from build123d import *

# Parameters (mm, degrees)
EXTRUDE_1_DEPTH     = 48
SKETCH_3_W          = 2
SKETCH_3_H          = 3.503465233
EXTRUDE_2_DEPTH     = 0.5
SKETCH_4_W          = 2
SKETCH_4_H          = 3.503465233
EXTRUDE_3_DEPTH     = 0.5
SKETCH_7_W          = 0.5
SKETCH_7_H          = 3.503465233
CUT_EXTRUDE_2_DEPTH = 66.5
SKETCH_10_W         = 2
SKETCH_10_H         = 0.5
CUT_EXTRUDE_3_DEPTH = 66.5
SKETCH_13_W         = 0.5
SKETCH_13_H         = 2
SKETCH_16_W         = 0.5
SKETCH_16_H         = 2


with BuildPart() as part:
    # Эскиз1 → Бобышка-Вытянуть1 (new body)
    with BuildSketch(Plane.XY):
        with BuildLine():
            Line((0.5, 0), (0.5, 25.5))
            ThreePointArc((0.5, 25.5), (0.646446609, 25.853553391), (1, 26))
            Line((1, 26), (18.5, 26))
            ThreePointArc((18.5, 26), (18.853553391, 25.853553391), (19, 25.5))
            Line((19, 25.5), (19, 0))
            Line((19, 0), (19.5, 0))
            Line((19.5, 0), (19.5, 25.5))
            ThreePointArc((19.5, 25.5), (19.207106781, 26.207106781), (18.5, 26.5))
            Line((18.5, 26.5), (1, 26.5))
            ThreePointArc((1, 26.5), (0.292893219, 26.207106781), (0, 25.5))
            Line((0, 25.5), (0, 0))
            Line((0, 0), (0.5, 0))
        make_face()
    extrude(amount=EXTRUDE_1_DEPTH)

    # Эскиз3 → Бобышка-Вытянуть2 (add)
    with BuildSketch(Plane.ZY):
        with Locations((45, -1.751732617)):
            Rectangle(SKETCH_3_W, SKETCH_3_H)
        with Locations((3, -1.751732617)):
            Rectangle(SKETCH_3_W, SKETCH_3_H)
    extrude(amount=-EXTRUDE_2_DEPTH)

    # Эскиз4 → Бобышка-Вытянуть3 (add)
    with BuildSketch(Plane(origin=(19.5, 0, 0), x_dir=(0, 0, -1), z_dir=(1, 0, 0))):
        with Locations((-45, -1.751732617)):
            Rectangle(SKETCH_4_W, SKETCH_4_H)
        with Locations((-3, -1.751732617)):
            Rectangle(SKETCH_4_W, SKETCH_4_H)
    extrude(amount=-EXTRUDE_3_DEPTH)

    # Эскиз7 → Вырез-Вытянуть2 (cut)
    with BuildSketch(Plane.ZY):
        with Locations((45.75, -1.751732617)):
            Rectangle(SKETCH_7_W, SKETCH_7_H)
        with Locations((3.75, -1.751732617)):
            Rectangle(SKETCH_7_W, SKETCH_7_H)
        with Locations((44.25, -1.751732617)):
            Rectangle(SKETCH_7_W, SKETCH_7_H)
        with Locations((2.25, -1.751732617)):
            Rectangle(SKETCH_7_W, SKETCH_7_H)
    extrude(amount=-CUT_EXTRUDE_2_DEPTH, mode=Mode.SUBTRACT)

    # По траектории2: sweep along a path in Эскиз9
    with BuildLine(Plane.ZY) as sweep_2_path:
        Line((48, 24.75), (48.353553391, 25.103553391))
        ThreePointArc((48.353553391, 25.103553391), (48.461939766, 25.265765065), (48.5, 25.457106781))
        Line((48.5, 25.457106781), (48.5, 25.75))
        ThreePointArc((48.5, 25.75), (48.353553391, 26.103553391), (48, 26.25))
        Line((48, 26.25), (0, 26.25))
        ThreePointArc((0, 26.25), (-0.353553391, 26.103553391), (-0.5, 25.75))
        Line((-0.5, 25.75), (-0.5, 25.457106781))
        ThreePointArc((-0.5, 25.457106781), (-0.461939766, 25.265765065), (-0.353553391, 25.103553391))
        Line((-0.353553391, 25.103553391), (0, 24.75))
    # Эскиз10 → По траектории2 (sweep)
    with BuildSketch(Plane(origin=(0, 24.75, 48), x_dir=(1, 0, 0), z_dir=(0, 0.7071067811865477, 0.7071067811865475))):
        with Locations((9.75, 0)):
            Rectangle(SKETCH_10_W, SKETCH_10_H)
    sweep(path=sweep_2_path.line)

    # Эскиз14 → Вырез-Вытянуть3 (cut)
    with BuildSketch(Plane.ZY):
        Polygon((2.5, 0), (3.5, 0), (3.5, 3), (44.5, 3), (44.5, 0), (45.5, 0), (45.5, 3), (48, 3), (48, 0), (46.949999013, 0), (46.949999013, -4.072410454), (1.67699977, -4.072410454), (1.67699977, 0), (0, 0), (0, 3), (2.5, 3), align=None)
    extrude(amount=-CUT_EXTRUDE_3_DEPTH, mode=Mode.SUBTRACT)

    # По траектории3: sweep along a path in Эскиз11
    with BuildLine(Plane(origin=(0, 26.5, 0), x_dir=(1, 0, 0), z_dir=(0, 1, 0))) as sweep_3_path:
        Line((17.75, 0), (18.103553391, 0.353553391))
        ThreePointArc((18.103553391, 0.353553391), (18.265765065, 0.461939766), (18.457106781, 0.5))
        Line((18.457106781, 0.5), (18.75, 0.5))
        ThreePointArc((18.75, 0.5), (19.103553391, 0.353553391), (19.25, 0))
        Line((19.25, 0), (19.25, -48))
        ThreePointArc((19.25, -48), (19.103553391, -48.353553391), (18.75, -48.5))
        Line((18.75, -48.5), (18.457106781, -48.5))
        ThreePointArc((18.457106781, -48.5), (18.265765065, -48.461939766), (18.103553391, -48.353553391))
        Line((18.103553391, -48.353553391), (17.75, -48))
    # Эскиз13 → По траектории3 (sweep)
    with BuildSketch(Plane(origin=(17.75, 26.5, 0), x_dir=(0.7071067811865498, 0, 0.7071067811865454), z_dir=(-0.7071067811865454, 0, 0.7071067811865498))):
        with Locations((0, -13.25)):
            Rectangle(SKETCH_13_W, SKETCH_13_H)
    sweep(path=sweep_3_path.line)

    # По траектории4: sweep along a path in Эскиз15
    with BuildLine(Plane(origin=(0, 26.5, 0), x_dir=(1, 0, 0), z_dir=(0, 1, 0))) as sweep_4_path:
        Line((1.75, 0), (1.396446609, 0.353553391))
        ThreePointArc((1.396446609, 0.353553391), (1.234234935, 0.461939766), (1.042893219, 0.5))
        Line((1.042893219, 0.5), (0.75, 0.5))
        ThreePointArc((0.75, 0.5), (0.396446609, 0.353553391), (0.25, 0))
        Line((0.25, 0), (0.25, -48))
        ThreePointArc((0.25, -48), (0.396446609, -48.353553391), (0.75, -48.5))
        Line((0.75, -48.5), (1.042893219, -48.5))
        ThreePointArc((1.042893219, -48.5), (1.234234935, -48.461939766), (1.396446609, -48.353553391))
        Line((1.396446609, -48.353553391), (1.75, -48))
    # Эскиз16 → По траектории4 (sweep)
    with BuildSketch(Plane(origin=(1.75, 26.5, 48), x_dir=(-0.7071067811865488, 0, -0.7071067811865464), z_dir=(0.7071067811865464, 0, -0.7071067811865488))):
        with Locations((0, -13.25)):
            Rectangle(SKETCH_16_W, SKETCH_16_H)
    sweep(path=sweep_4_path.line)


solid = part.part
Can you work these out from the model? Positions are in its coordinate system, mm. A direction names the side the tool comes from. Round coordinates to 2 decimals unless told otherwise and drop trailing zeros. Write each loop counter-clockwise with the first axis right and the second up, starting at its lowest first coordinate (ties: lowest second). Pieces come first, ordered by that corner, then holes. Notation, with made-up numbers: M 6,-7 L 17,-7 A21 cw 17,15 Z; hole C 77.5,17 d4. An arc over 180 degrees is marked long. Use a Markdown table: item, result.
Item 1: Which directions (+Z, -Z, +X, -X, +Y, -Y) give clear straight access to the entire face, cutting with the end or side of a thin tool? Please do faces 1 (the face through (0.301, 26.215, 23.664)), 2 (the face through (19.3, 23.1, 0)), 3 (the face through (0.5, 13, 24)), 4 (the face through (19.3, 23.1, 48)).
Found:
| item | result |
|---|---|
| face 1 | +Z, -Z, -X, +Y |
| face 2 | -Z, +X, +Y |
| face 3 | -Y |
| face 4 | +Z, +X, +Y |
Item 2: If I drill on line 1 along X through (y, z) = (22.75, 35); line 2 along Y through (x, z) = (3.75, 20), over which ranges is the centre line in solid material (lowest first)? Write a range as [from, to].
Found:
| item | result |
|---|---|
| line 1 | x = [0, 0.5], [19, 19.5] |
| line 2 | y = [26, 26.5] |
Item 3: I want a section at A-A (y = 15.75). List the corners of the cut face in (x, z) for me, and give its area (3 significant figures).
Found:
| item | result |
|---|---|
| outline | M 0,0 L 0.5,0 L 0.5,48 L 0,48 Z; M 19,0 L 19.5,0 L 19.5,48 L 19,48 Z |
| area | 48.0 mm2 |
Item 4: I want a section at D-D (x = 12.5). List the corners of the cut face in (y, z) for me, and give its area (3 significant figures).
Found:
| item | result |
|---|---|
| outline | M 26,0 L 26.5,0 L 26.5,48 L 26,48 Z |
| area | 24.0 mm2 |
Item 5: For pin 1 Ø0.5 at (x, z) = (0.5, 48.5) entering from -Y; pin 2 Ø1 at (x, z) = (13.5, 33) entering from -Y; pin 3 Ø7 at (x, y) = (6, 19) entering from +Z; pin 4 Ø0.6 at (x, z) = (0.5, 47.5) entering from -Y, each with a flat end and sliding along its axis, tell me the tip position at first contact or that it passes through.
Found:
| item | result |
|---|---|
| pin 1 | stops at y = 12.25 |
| pin 2 | stops at y = 26 |
| pin 3 | passes through |
| pin 4 | stops at y = 3 |
Item 6: I want a section at B-B (y = 2.25). List the corners of the cut face in (x, z) for me.
Found:
| item | result |
|---|---|
| outline | M 0,2.5 L 0.5,2.5 L 0.5,3.5 L 0,3.5 Z; M 0,44.5 L 0.5,44.5 L 0.5,45.5 L 0,45.5 Z; M 19,2.5 L 19.5,2.5 L 19.5,3.5 L 19,3.5 Z; M 19,44.5 L 19.5,44.5 L 19.5,45.5 L 19,45.5 Z |
Item 7: I want a section at C-C (z = 44). List the corners of the cut face in (x, y) for me, and give its area (3 significant figures).
Found:
| item | result |
|---|---|
| outline | M 0,3 L 0.5,3 L 0.5,25.5 A0.5 cw 1,26 L 18.5,26 A0.5 cw 19,25.5 L 19,3 L 19.5,3 L 19.5,25.5 A1 ccw 18.5,26.5 L 1,26.5 A1 ccw 0,25.5 Z |
| area | 32.4 mm2 |
Item 8: We'd pull the mould along X, two halves only. Please class faces 5 (the face through (10, 26.5, 24)), 6 (the face through (10, 26, 24)), 7 (the face through (0, 13, 24)), 8 (the face through (19.215, 26.199, 23.664)): released by +X, released by -X, zero draft, split by the parting line, or undercut.
Found:
| item | result |
|---|---|
| face 5 | zero draft |
| face 6 | undercut |
| face 7 | released by -X |
| face 8 | released by +X |
